Verification items for the finished model (mm, model axes). Face numbers are marked on the shaded views. A direction names the side the tool comes from. Round coordinates to 2 decimals unless told otherwise and drop trailing zeros. Write each loop counter-clockwise with the first axis right and the second up, starting at its lowest first coordinate (ties: lowest second). Pieces come first, ordered by that corner, then holes. Notation, with made-up numbers: M 26.25,-9 L 66.25,-9 A16 cw 66.25,6 Z; hole C 68.25,15 d8. An arc over 180 degrees is marked long. One line per item, written item: value. Start each with the question number.
from build123d import *

# Parameters (mm, degrees)
EXTRUDE_THIN1_DEPTH      = 15
EXTRUDE_THIN1_DEPTH_BACK = 15
BOSS_EXTRUDE1_DEPTH      = 1
SKETCH3_R                = 3
SKETCH3_R_2              = 1
BOSS_EXTRUDE2_DEPTH      = 5
BOSS_EXTRUDE3_DEPTH      = 2
BOSS_EXTRUDE4_START      = -30
BOSS_EXTRUDE4_DEPTH      = 2
SKETCH5_W                = 34.167254682
SKETCH5_H                = 5.095662734
BOSS_EXTRUDE5_DEPTH      = 2
BOSS_EXTRUDE6_START      = -84
SKETCH5_3_W              = 34.167254682
SKETCH5_3_H              = 5.095662734
BOSS_EXTRUDE6_DEPTH      = 2
CUT_EXTRUDE1_DEPTH       = 85


with BuildPart() as part:
    # Sketch1 → Extrude-Thin1 (new body, two sides)
    with BuildSketch(Plane(origin=(0, 0, 0), x_dir=(1, 0, 0), z_dir=(0, 1, 0))) as extrude_thin1_sk:
        with BuildLine():
            Line((-42, 22), (-42, -22))
            ThreePointArc((-42, -22), (-40.535533906, -25.535533906), (-37, -27))
            Line((-37, -27), (37, -27))
            ThreePointArc((37, -27), (40.535533906, -25.535533906), (42, -22))
            Line((42, -22), (42, 22))
            ThreePointArc((42, 22), (40.535533906, 25.535533906), (37, 27))
            Line((37, 27), (-37, 27))
            ThreePointArc((-37, 27), (-40.535533906, 25.535533906), (-42, 22))
        make_face()
        with BuildLine():
            Line((-40, 22), (-40, -22))
            ThreePointArc((-40, -22), (-39.121320344, -24.121320344), (-37, -25))
            Line((-37, -25), (37, -25))
            ThreePointArc((37, -25), (39.121320344, -24.121320344), (40, -22))
            Line((40, -22), (40, 22))
            ThreePointArc((40, 22), (39.121320344, 24.121320344), (37, 25))
            Line((37, 25), (-37, 25))
            ThreePointArc((-37, 25), (-39.121320344, 24.121320344), (-40, 22))
        make_face(mode=Mode.SUBTRACT)
    extrude(amount=EXTRUDE_THIN1_DEPTH)
    extrude(extrude_thin1_sk.sketch, amount=-EXTRUDE_THIN1_DEPTH_BACK)

    # Sketch1<2> → Boss-Extrude1 (add)
    with BuildSketch(Plane(origin=(0, 0, 0), x_dir=(1, 0, 0), z_dir=(0, 1, 0))):
        with BuildLine():
            Line((-37, -25), (37, -25))
            ThreePointArc((37, -25), (39.121320344, -24.121320344), (40, -22))
            Line((40, -22), (40, 22))
            ThreePointArc((40, 22), (39.121320344, 24.121320344), (37, 25))
            Line((37, 25), (-37, 25))
            ThreePointArc((-37, 25), (-39.121320344, 24.121320344), (-40, 22))
            Line((-40, 22), (-40, -22))
            ThreePointArc((-40, -22), (-39.121320344, -24.121320344), (-37, -25))
        make_face()
    extrude(amount=BOSS_EXTRUDE1_DEPTH)

    # Sketch3 → Boss-Extrude2 (add)
    with BuildSketch(Plane(origin=(0, 1, 0), x_dir=(1, 0, 0), z_dir=(0, 1, 0))):
        with Locations((-30, 15)):
            Circle(SKETCH3_R)
        with Locations((-30, 15)):
            Circle(SKETCH3_R_2, mode=Mode.SUBTRACT)
        with Locations((30, 15)):
            Circle(SKETCH3_R)
        with Locations((30, 15)):
            Circle(SKETCH3_R_2, mode=Mode.SUBTRACT)
        with Locations((30, -15)):
            Circle(SKETCH3_R)
        with Locations((30, -15)):
            Circle(SKETCH3_R_2, mode=Mode.SUBTRACT)
        with Locations((-30, -15)):
            Circle(SKETCH3_R)
        with Locations((-30, -15)):
            Circle(SKETCH3_R_2, mode=Mode.SUBTRACT)
    extrude(amount=BOSS_EXTRUDE2_DEPTH)

    # Sketch4 → Boss-Extrude3 (add)
    with BuildSketch(Plane(origin=(0, 15, 0), x_dir=(1, 0, 0), z_dir=(0, 1, 0))):
        with BuildLine():
            Line((-35, 25), (-35, 27))
            Line((-35, 27), (-37, 27))
            ThreePointArc((-37, 27), (-40.535533906, 25.535533906), (-42, 22))
            Line((-42, 22), (-42, -22))
            ThreePointArc((-42, -22), (-40.535533906, -25.535533906), (-37, -27))
            Line((-37, -27), (-35, -27))
            Line((-35, -27), (-35, -25))
            Line((-35, -25), (-37, -25))
            ThreePointArc((-37, -25), (-39.121320344, -24.121320344), (-40, -22))
            Line((-40, -22), (-40, 22))
            ThreePointArc((-40, 22), (-39.121320344, 24.121320344), (-37, 25))
            Line((-37, 25), (-35, 25))
        make_face()
        with BuildLine():
            Line((-35, -25), (-35, 25))
            Line((-35, 25), (-37, 25))
            ThreePointArc((-37, 25), (-39.121320344, 24.121320344), (-40, 22))
            Line((-40, 22), (-40, -22))
            ThreePointArc((-40, -22), (-39.121320344, -24.121320344), (-37, -25))
            Line((-37, -25), (-35, -25))
        make_face()
        with BuildLine():
            Line((37, 25), (35, 25))
            Line((35, 25), (35, 3))
            Line((35, 3), (37, 3))
            Line((37, 3), (37, -3))
            Line((37, -3), (35, -3))
            Line((35, -3), (35, -25))
            Line((35, -25), (37, -25))
            ThreePointArc((37, -25), (39.121320344, -24.121320344), (40, -22))
            Line((40, -22), (40, 22))
            ThreePointArc((40, 22), (39.121320344, 24.121320344), (37, 25))
        make_face()
        with BuildLine():
            Line((37, 27), (35, 27))
            Line((35, 27), (35, 25))
            Line((35, 25), (37, 25))
            ThreePointArc((37, 25), (39.121320344, 24.121320344), (40, 22))
            Line((40, 22), (40, -22))
            ThreePointArc((40, -22), (39.121320344, -24.121320344), (37, -25))
            Line((37, -25), (35, -25))
            Line((35, -25), (35, -27))
            Line((35, -27), (37, -27))
            ThreePointArc((37, -27), (40.535533906, -25.535533906), (42, -22))
            Line((42, -22), (42, 22))
            ThreePointArc((42, 22), (40.535533906, 25.535533906), (37, 27))
        make_face()
    extrude(amount=BOSS_EXTRUDE3_DEPTH)

    # Sketch4<3> → Boss-Extrude4 (add)
    with BuildSketch(Plane(origin=(0, 15, 0), x_dir=(1, 0, 0), z_dir=(0, 1, 0)).offset(BOSS_EXTRUDE4_START)):
        with BuildLine():
            Line((-35, -25), (-35, 25))
            Line((-35, 25), (-37, 25))
            ThreePointArc((-37, 25), (-39.121320344, 24.121320344), (-40, 22))
            Line((-40, 22), (-40, -22))
            ThreePointArc((-40, -22), (-39.121320344, -24.121320344), (-37, -25))
            Line((-37, -25), (-35, -25))
        make_face()
        with BuildLine():
            Line((-35, 25), (-35, 27))
            Line((-35, 27), (-37, 27))
            ThreePointArc((-37, 27), (-40.535533906, 25.535533906), (-42, 22))
            Line((-42, 22), (-42, -22))
            ThreePointArc((-42, -22), (-40.535533906, -25.535533906), (-37, -27))
            Line((-37, -27), (-35, -27))
            Line((-35, -27), (-35, -25))
            Line((-35, -25), (-37, -25))
            ThreePointArc((-37, -25), (-39.121320344, -24.121320344), (-40, -22))
            Line((-40, -22), (-40, 22))
            ThreePointArc((-40, 22), (-39.121320344, 24.121320344), (-37, 25))
            Line((-37, 25), (-35, 25))
        make_face()
        with BuildLine():
            Line((37, 25), (35, 25))
            Line((35, 25), (35, 3))
            Line((35, 3), (37, 3))
            Line((37, 3), (37, -3))
            Line((37, -3), (35, -3))
            Line((35, -3), (35, -25))
            Line((35, -25), (37, -25))
            ThreePointArc((37, -25), (39.121320344, -24.121320344), (40, -22))
            Line((40, -22), (40, 22))
            ThreePointArc((40, 22), (39.121320344, 24.121320344), (37, 25))
        make_face()
        with BuildLine():
            Line((37, 27), (35, 27))
            Line((35, 27), (35, 25))
            Line((35, 25), (37, 25))
            ThreePointArc((37, 25), (39.121320344, 24.121320344), (40, 22))
            Line((40, 22), (40, -22))
            ThreePointArc((40, -22), (39.121320344, -24.121320344), (37, -25))
            Line((37, -25), (35, -25))
            Line((35, -25), (35, -27))
            Line((35, -27), (37, -27))
            ThreePointArc((37, -27), (40.535533906, -25.535533906), (42, -22))
            Line((42, -22), (42, 22))
            ThreePointArc((42, 22), (40.535533906, 25.535533906), (37, 27))
        make_face()
    extrude(amount=-BOSS_EXTRUDE4_DEPTH)

    # Sketch5 → Boss-Extrude5 (add)
    with BuildSketch(Plane.ZY.offset(42)):
        Polygon((21.083627341, -7.904337266), (-21.083627341, -7.904337266), (-21.083627341, -17), (-17.083627341, -17), (-17.083627341, -11.904337266), (17.083627341, -11.904337266), (17.083627341, -17), (21.083627341, -17), align=None)
        Polygon((-17.083627341, -17), (-21.083627341, -17), (-21.083627341, -26.095662734), (21.083627341, -26.095662734), (21.083627341, -17), (17.083627341, -17), (17.083627341, -22.095662734), (-17.083627341, -22.095662734), align=None)
        with Locations((0, -14.452168633)):
            Rectangle(SKETCH5_W, SKETCH5_H)
    extrude(amount=-BOSS_EXTRUDE5_DEPTH)

    # Sketch5<3> → Boss-Extrude6 (add)
    with BuildSketch(Plane.ZY.offset(42).offset(BOSS_EXTRUDE6_START)):
        Polygon((21.083627341, -7.904337266), (-21.083627341, -7.904337266), (-21.083627341, -17), (-17.083627341, -17), (-17.083627341, -11.904337266), (17.083627341, -11.904337266), (17.083627341, -17), (21.083627341, -17), align=None)
        with Locations((0, -14.452168633)):
            Rectangle(SKETCH5_3_W, SKETCH5_3_H)
        Polygon((-17.083627341, -17), (-21.083627341, -17), (-21.083627341, -26.095662734), (21.083627341, -26.095662734), (21.083627341, -17), (17.083627341, -17), (17.083627341, -22.095662734), (-17.083627341, -22.095662734), align=None)
    extrude(amount=BOSS_EXTRUDE6_DEPTH)

    # Sketch7 → Cut-Extrude1 (cut, through all)
    with BuildSketch(Plane(origin=(42, 0, 0), x_dir=(0, 0, -1), z_dir=(1, 0, 0))):
        with BuildLine():
            Line((-8.338334794, 14), (8.338334794, 14))
            ThreePointArc((8.338334794, 14), (10.338334794, 12), (8.338334794, 10))
            Line((8.338334794, 10), (-8.338334794, 10))
            ThreePointArc((-8.338334794, 10), (-10.338334794, 12), (-8.338334794, 14))
        make_face()
    extrude(amount=-CUT_EXTRUDE1_DEPTH, mode=Mode.SUBTRACT)


solid = part.part
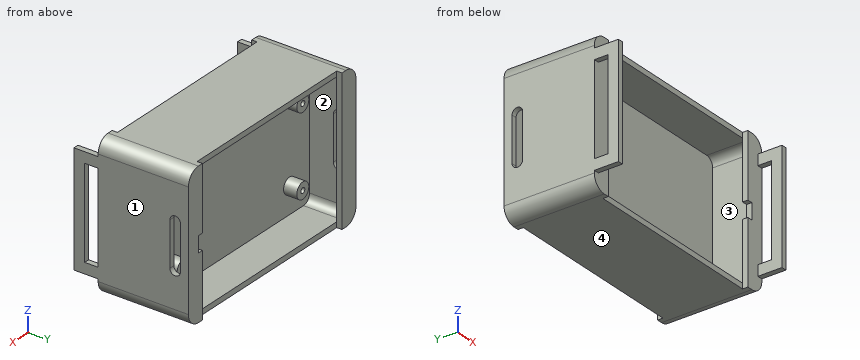
1) Cross-section at B-B (y = 5). State how many separate pieces and enclosed holes the cut face has, then the cut area to 3 significant figures.
2) Cross-section at A-A (y = -2). Record the boundary of the cut face in (x, z), then the cut area to 3 significant figures.
3) Thickness scan on line 1 (Z direction, x = 30, y = 3); line 2 (X direction, y = 2.85, z = 15); line 3 (Y direction, x = -36.5, z = 16.5). Record the ranges inside material, lowest first.
4) Gauge pin test, flat ends, axial feed: pin 1 Ø4 at (x, z) = (31.5, 2.5) entering from -Y; pin 2 Ø1.6 at (x, y) = (41, -18.5) entering from -Z; pin 3 Ø15 at (x, z) = (2.5, 5) entering from +Y. Record the tip position at first contact, or that the pin passes through.
5) Mould release check, pull along Y, two halves, no side actions. Record for the marked faces 3 and 4: pulls with the +Y half, pulls with the -Y half, needs draft (parallel to the pull), parting line crosses it, or undercut.
6) Access from +Z, -Z, +X, -X, +Y, -Y to the whole of each face (thin tool, end or side, straight path). Record for the marked faces 1 and 2.
7) Cross-section at C-C (x = 36). Record the boundary of the cut face in (y, z).
Results below:
1. separate pieces: 5
1. enclosed holes: 5
1. area: 623 mm²
2. outline: M -42,-22 A5 ccw -37,-27 L 37,-27 A5 ccw 42,-22 L 42,22 A5 ccw 37,27 L -37,27 A5 ccw -42,22 Z; hole M -40,-22 A3 ccw -37,-25 L 37,-25 A3 ccw 40,-22 L 40,22 A3 ccw 37,25 L -37,25 A3 ccw -40,22 Z
2. area: 522 mm²
3. line 1: z = -27 to -25, -18 to -16, -14 to -12, 12 to 14, 16 to 18, 25 to 27
3. line 2: x = -42 to -40, -33 to -31, -29 to -27, 27 to 29, 31 to 33, 40 to 42
3. line 3: y = -17 to -15, 0 to 1, 15 to 17
4. pin 1: stops at y = 0
4. pin 2: stops at z = -21.08
4. pin 3: stops at y = 1
5. face 3: undercut
5. face 4: needs draft
6. face 1: +Z, -Z, +X, +Y, -Y
6. face 2: none
7. outline: M -17,-27 L 17,-27 L 17,-3 L 15,-3 L 15,-25 L 1,-25 L 1,25 L 15,25 L 15,3 L 17,3 L 17,27 L -17,27 L -17,3 L -15,3 L -15,25 L 0,25 L 0,-25 L -15,-25 L -15,-3 L -17,-3 Z
